Read the model definition and answer for the solid it produces. Units are mm, in the model's axes. Face numbers are marked on the shaded views. A direction names the side the tool comes from. Give positions to 0.01 mm unless a question says otherwise; leave off trailing zeros. Write each loop counter-clockwise with the first axis right and the second up, starting at its lowest first coordinate (ties: lowest second). Pieces come first, ordered by that corner, then holes. Notation, with made-up numbers: (-23, -21.75) -> (18, -21.75) arc R14 cw to (18, -1.75) -> close; hole circle Ø3 at (-18.5, -20). An arc over 180 degrees is marked (long way). Answer as CSV lines item,"result". Start each with the question number.
1. The part is cut by section D-D, the plane y = -186. Determine the outline of the cut face in (x, z), and give its area (3 significant figures).
2. Given pin 1 (6 mm diameter, centred on y = -93.5, z = 41.5, fed in from +X); pin 2 (14 mm diameter, centred on x = -168, y = 9, fed in from +Z); pin 3 (12 mm diameter, centred on x = -104, y = 27, fed in from -Z); pin 4 (12 mm diameter, centred on y = 39, z = -192.5, fed in from +X), each flat-ended and moving along its own axis, determine where each tip first touches the part or whether it passes through.
3. The part is cut by section A-A, the plane z = -238. Determine the outline of the cut face in (x, y).
4. The part is cut by section C-C, the plane x = -201. Determine the outline of the cut face in (y, z), and give its area (3 significant figures).
5. A tool of negligible diameter and unlimited length cuts with its end or side. For the marked faces 1, 2 and 3, from which of +Z, -Z, +X, -X, +Y, -Y can it reach the whole face along a straight path? Write none if from no direction.
6. The part is cut by section B-B, the plane z = -18. Determine the outline of the cut face in (x, y).
7. For a pull along Z with two mould halves and no side action, classify the marked faces 4, 5 and 6 as pulls with the +Z half, pulls with the -Z half, needs draft (parallel to the pull), parting line crosses it, or undercut.
8. Find the intervals of material crossed by line 1 (Z direction, x = 0, y = 138); line 2 (Y direction, x = 0, z = 68); line 3 (X direction, y = -122.5, z = -160.5), in increasing order.
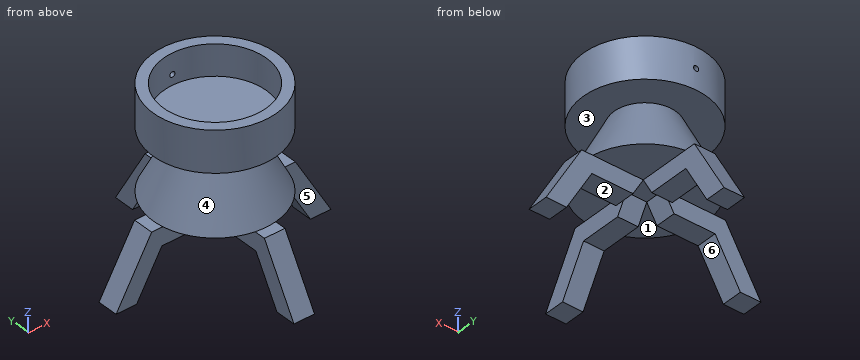
from build123d import *

# Parameters (mm, degrees)
F0_R      = 127
F1_DEPTH  = 25.4
F0_R_2    = 152.4
F2_DEPTH  = 101.6
F3_R      = 6.35
F4_DEPTH  = 152.401
F5_R      = 76.2
F7_R      = 152.4
F10_DEPTH = 25.4
F12_DEPTH = 25.4


with BuildPart() as f1:
    # F0 (on Top) → F1 (new body)
    with BuildSketch(Plane.XY):
        Circle(F0_R)
    extrude(amount=F1_DEPTH)

    # F0 (on Top) → F2 (join)
    with BuildSketch(Plane.XY):
        Circle(F0_R_2)
        Circle(F0_R, mode=Mode.SUBTRACT)
    extrude(amount=F2_DEPTH)

    # F3 (on Front) → F4 (cut, through all)
    with BuildSketch(Plane.XZ):
        with Locations((0, 50.8)):
            Circle(F3_R)
    extrude(amount=-F4_DEPTH, mode=Mode.SUBTRACT)

    # F5 (on face) → F8 section 0
    with BuildSketch(Plane(origin=(0, 0, 0), x_dir=(1, 0, 0), z_dir=(0, 0, -1))):
        Circle(F5_R)
    # F7 (on offset) → F8 section 1
    with BuildSketch(Plane(origin=(0, 0, -152.4), x_dir=(1, 0, 0), z_dir=(0, 0, -1))):
        Circle(F7_R)
    loft()

    # F9 (on Front) → F10 (join, symmetric)
    with BuildSketch(Plane.XZ):
        Polygon((-50.8, -196.394091), (-25.4, -152.4), (-152.4, -152.4), (-177.8, -152.4), (-265.788181, -304.8), (-214.988181, -304.8), (-152.4, -196.394091), align=None)
        Polygon((177.8, -152.4), (152.4, -152.4), (152.4, -196.394091), (214.988181, -304.8), (265.788181, -304.8), align=None)
        Polygon((152.4, -152.4), (25.4, -152.4), (50.8, -196.394091), (152.4, -196.394091), align=None)
    extrude(amount=F10_DEPTH, both=True)

    # F11 (on Right) → F12 (join, symmetric)
    with BuildSketch(Plane.YZ):
        Polygon((152.4, -152.4), (25.4, -152.4), (50.8, -196.394091), (152.4, -196.394091), align=None)
        Polygon((-50.8, -196.394091), (-25.4, -152.4), (-152.4, -152.4), (-152.4, -196.394091), align=None)
        Polygon((177.8, -152.4), (152.4, -152.4), (152.4, -196.394091), (214.988181, -304.8), (265.788181, -304.8), align=None)
        Polygon((-152.4, -196.394091), (-152.4, -152.4), (-177.8, -152.4), (-265.788181, -304.8), (-214.988181, -304.8), align=None)
    extrude(amount=F12_DEPTH, both=True)


solid = f1.part
Results found:
1,outline,"(-25.4, -254.59) -> (25.4, -254.59) -> (25.4, -166.6) -> (-25.4, -166.6) -> close"
1,area,"4,470 mm²"
2,pin 1,"stops at x = 122.62"
2,pin 2,"stops at z = -152.4"
2,pin 3,"stops at z = -196.39"
2,pin 4,"passes through"
3,outline,"(-227.22, -25.4) -> (-176.42, -25.4) -> (-176.42, 25.4) -> (-227.22, 25.4) -> close; (-25.4, -227.22) -> (25.4, -227.22) -> (25.4, -176.42) -> (-25.4, -176.42) -> close; (-25.4, 176.42) -> (25.4, 176.42) -> (25.4, 227.22) -> (-25.4, 227.22) -> close; (176.42, -25.4) -> (227.22, -25.4) -> (227.22, 25.4) -> (176.42, 25.4) -> close"
4,outline,"(-25.4, -280.57) -> (25.4, -280.57) -> (25.4, -192.58) -> (-25.4, -192.58) -> close"
4,area,"4,470 mm²"
5,face 1,"-Z, -X, -Y"
5,face 2,"-Z, +Y, -Y"
5,face 3,"none"
6,outline,"circle Ø170.4 at (0, 0)"
7,face 4,"undercut"
7,face 5,"needs draft"
7,face 6,"pulls with the -Z half"
8,line 1,"z = -196.39 to -123.6, 0 to 44.45, 57.15 to 101.6"
8,line 2,"y = -152.4 to -127, 127 to 152.4"
8,line 3,"x = -25.4 to 25.4"
